Build history of the part. All positions in model axes, mm. Face numbers are marked on the shaded views. Give positions to 0.01 mm unless a question says otherwise; leave off trailing zeros. Order: outer loops, then holes, each group sorted by start corner. A loop starts at its lowest first (then second) coordinate and runs counter-clockwise, first axis right, second up. Notation, with made-up numbers: (51, 11.5) -> (57, 11.5) arc R26 ccw to (57, 48.5) -> close; hole circle Ø1 at (-4.5, 30.5). An arc over 180 degrees is marked (long way). One line per question, with ' | ' between items. Start each with the question number.
(1) Drill centre lines: L1, parallel to Y at x = 59.25, z = -5.5; L2, parallel to Z at x = 60.75, y = 159.25; L3, parallel to Z at x = 61.3, y = 160. Where is each one in solid material? Low to high. Write a range as from..to.
(2) Cut at B-B (y = 168). Give the cut face in (x, z), then the cut area to 3 significant figures.
(3) Cut at C-C (z = -7). Give the cut face in (x, y), then the cut area to 3 significant figures.
(4) Pull direction Y, two halves, no side cores. Call the marked faces 1, 2, 3 and 4: +Y half, -Y half, draft (parallel to the pull), parting line (faces both ways), or undercut.
(5) Pin check, flat tips, straight feed: pin 1 Ø1.2 at (x, y) = (61, 161) entering from -Z; pin 2 Ø1.8 at (x, z) = (60.5, 14) entering from +Y; pin 3 Ø1.5 at (x, z) = (60, -6.5) entering from +Y; pin 4 Ø9.5 at (y, z) = (160.5, -0.5) entering from -X. Stop position of each tip, or through.
(6) Cut at A-A (x = 62.6). Give the number of separate pieces and of enclosed holes in the cut face, then the cut area to 3 significant figures.
(7) Cut at D-D (y = 161.5). Give the cut face in (x, z), then the cut area to 3 significant figures.
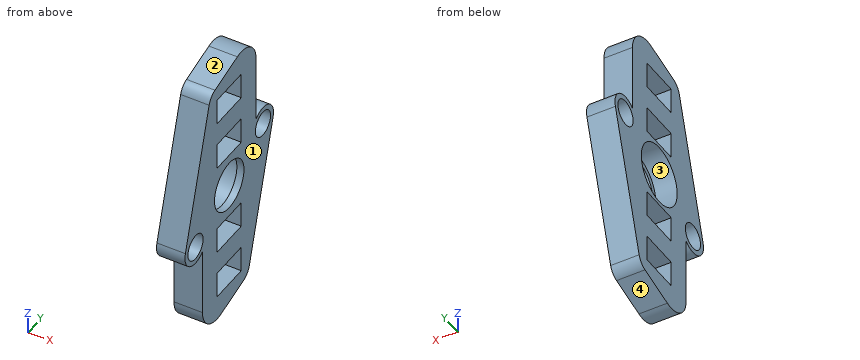
from build123d import *

# Parameters (mm, degrees)
SKETCH171_R     = 4.25
PAD127009_DEPTH = 3
SKETCH147_R     = 3.5
SKETCH147_R_2   = 1.8
SKETCH147_W     = 5.7
SKETCH147_H     = 3.7
PAD115_DEPTH    = 4


with BuildPart() as bearingcutout:
    # Sketch171 → Pad127009 (new body)
    with BuildSketch(Plane(origin=(59, 160, 0), x_dir=(0, 1, 0), z_dir=(1, 0, 0))):
        Circle(SKETCH171_R)
    extrude(amount=PAD127009_DEPTH)


with BuildPart() as wheelbearingbase:
    # Sketch147 → Pad115 (new body)
    with BuildSketch(Plane(origin=(59, 160, 0), x_dir=(0, 1, 0), z_dir=(1, 0, 0))):
        with BuildLine():
            ThreePointArc((10.40007, 3.300239), (9.342414, 6.10901), (6.35, 5.878164))
            Line((6.35, 5.878164), (6.35, 15.45))
            ThreePointArc((6.35, 15.45), (4.974419, 18.231518), (1.928947, 18.826635))
            Line((-3.376316, 17.379506), (1.928947, 18.826635))
            ThreePointArc((-3.376316, 17.379506), (-4.251863, 16.876457), (-4.770061, 16.00979))
            Line((-10.40007, -3.300239), (-4.770061, 16.00979))
            ThreePointArc((-10.40007, -3.300239), (-9.342414, -6.10901), (-6.35, -5.878164))
            Line((-6.35, -5.878164), (-6.35, -15.45))
            ThreePointArc((-6.35, -15.45), (-4.974419, -18.231518), (-1.928947, -18.826635))
            Line((-1.928947, -18.826635), (3.376315, -17.379506))
            ThreePointArc((3.376315, -17.379506), (4.251856, -16.876464), (4.770056, -16.009808))
            Line((10.40007, 3.300239), (4.770056, -16.009808))
        make_face()
        Circle(SKETCH147_R, mode=Mode.SUBTRACT)
        with Locations((-8, -4)):
            Circle(SKETCH147_R_2, mode=Mode.SUBTRACT)
        with Locations((8, 4)):
            Circle(SKETCH147_R_2, mode=Mode.SUBTRACT)
        with Locations((0, 6.6)):
            Rectangle(SKETCH147_W, SKETCH147_H, mode=Mode.SUBTRACT)
        with Locations((0, -13.6)):
            Rectangle(SKETCH147_W, SKETCH147_H, mode=Mode.SUBTRACT)
        with Locations((0, 13.6)):
            Rectangle(SKETCH147_W, SKETCH147_H, mode=Mode.SUBTRACT)
        with Locations((0, -6.6)):
            Rectangle(SKETCH147_W, SKETCH147_H, mode=Mode.SUBTRACT)
    extrude(amount=PAD115_DEPTH)

    # Cut007019018: cut BearingCutout
    add(bearingcutout.part, mode=Mode.SUBTRACT)


solid = wheelbearingbase.part
Result set:
1) L1: y = 150..151.01, 152.99..157.15, 162.85..167.83 | L2: z = -18.51..-15.45, -11.75..-8.45, -4.75..-4.18, 4.18..4.75, 8.45..11.75, 15.45..18.1 | L3: z = -18.3..-15.45, -11.75..-8.45, -4.75..-4.25, 4.25..4.75, 8.45..11.75, 15.45..18.3
2) outline: (59, -4.93) -> (63, -4.93) -> (63, 2.2) -> (59, 2.2) -> close; (59, 5.8) -> (63, 5.8) -> (63, 6.5) -> (59, 6.5) -> close | area: 31.3 mm2
3) outline: (59, 153.65) -> (63, 153.65) -> (63, 157.15) -> (59, 157.15) -> close; (59, 162.85) -> (63, 162.85) -> (63, 167.4) -> (59, 167.4) -> close | area: 32.2 mm2
4) face 1: draft | face 2: -Y half | face 3: undercut | face 4: +Y half
5) pin 1: stops at z = -18.19 | pin 2: stops at y = 166.35 | pin 3: stops at y = 167.76 | pin 4: stops at x = 59
6) separate pieces: 1 | enclosed holes: 7 | area: 380 mm2
7) outline: (59, -17.89) -> (63, -17.89) -> (63, -15.45) -> (59, -15.45) -> close; (59, -11.75) -> (63, -11.75) -> (63, -8.45) -> (59, -8.45) -> close; (59, -4.75) -> (63, -4.75) -> (63, -3.16) -> (62, -3.16) -> (62, -3.98) -> (59, -3.98) -> close; (59, 3.98) -> (62, 3.98) -> (62, 3.16) -> (63, 3.16) -> (63, 4.75) -> (59, 4.75) -> close; (59, 8.45) -> (63, 8.45) -> (63, 11.75) -> (59, 11.75) -> close; (59, 15.45) -> (63, 15.45) -> (63, 18.71) -> (59, 18.71) -> close | area: 57.0 mm2
